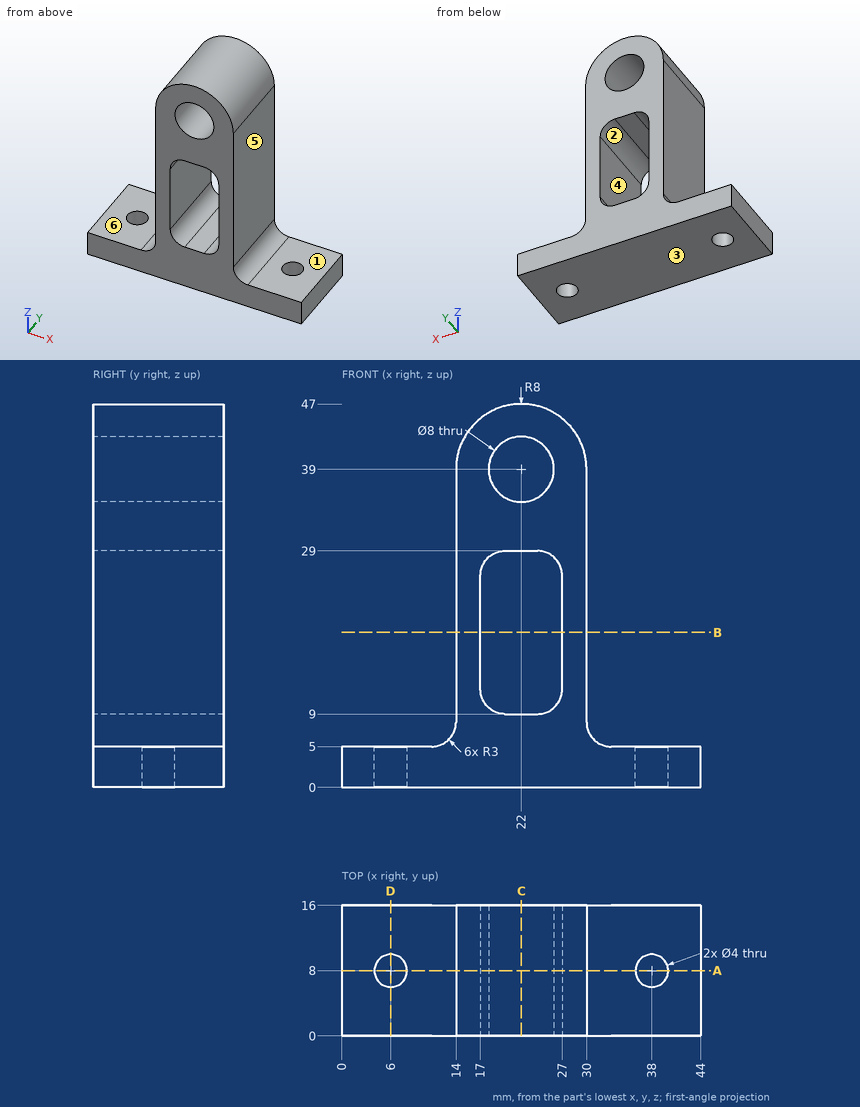
Geometry: see drawing. Coordinates: mm, zero at the bounding-box minimum. A direction names the side the tool comes from. Coordinates: 2 decimals unless noted, no trailing zeros. Loops run counter-clockwise (first coordinate to the right, second up) from the corner with the lowest first, then second, coordinate; pieces in that order, holes last.
(1) Section D-D on x = 6. Return the cut outline in (y, z), then the cut area to 3 significant figures.
(2) First-contact query: pin 1 Ø2 at (x, y) = (34.5, 8) entering from +Z; pin 2 Ø8 at (x, y) = (32.5, 10) entering from +Z; pin 3 Ø7 at (y, z) = (4, 20) entering from -X. Flat tips, straight axial feed; report the tip coordinate or a pass-through.
(3) Section A-A on y = 8. Return the cut outline in (x, z).
(4) Set-up query: the marked faces 4, 5 and 6. Return all of +Z, -Z, +X, -X, +Y, -Y with unobstructed straight access to the full face (end or side cutting, diameter ignored); none if empty.
(5) Pull-direction query (Z, two-part tool) for the marked faces 1, 2 and 3; classes: released by +Z, released by -Z, zero draft, split by the parting line, or undercut.
(6) Section C-C on x = 22. Return the cut outline in (y, z).
(7) Material intervals for probe 1 along X at (y, z) = (8, 2.9); probe 2 along Z at (x, y) = (22, 10.75); probe 3 along X at (y, z) = (9.75, 14), sorted ascending.
(8) Section B-B on z = 19. Return the cut outline in (x, y).
Data:
1. outline: (0, 0) - (6, 0) - (6, 5) - (0, 5) - close; (10, 0) - (16, 0) - (16, 5) - (10, 5) - close
1. area: 60.0 mm2
2. pin 1: stops at z = 5
2. pin 2: stops at z = 43.66
2. pin 3: stops at x = 14
3. outline: (0, 0) - (4, 0) - (4, 5) - (0, 5) - close; (8, 0) - (36, 0) - (36, 5) - (33, 5) arc R3 cw to (30, 8) - (30, 39) arc R8 ccw to (14, 39) - (14, 8) arc R3 cw to (11, 5) - (8, 5) - close; (40, 0) - (44, 0) - (44, 5) - (40, 5) - close; hole (17, 12) arc R3 ccw to (20, 9) - (24, 9) arc R3 ccw to (27, 12) - (27, 26) arc R3 ccw to (24, 29) - (20, 29) arc R3 ccw to (17, 26) - close; hole circle Ø8 at (22, 39)
4. face 4: +Y, -Y
4. face 5: +Z, +X, +Y, -Y
4. face 6: +Z, -X, +Y, -Y
5. face 1: released by +Z
5. face 2: undercut
5. face 3: released by -Z
6. outline: (0, 0) - (16, 0) - (16, 9) - (0, 9) - close; (0, 29) - (16, 29) - (16, 35) - (0, 35) - close; (0, 43) - (16, 43) - (16, 47) - (0, 47) - close
7. probe 1: x = 0 to 4, 8 to 36, 40 to 44
7. probe 2: z = 0 to 9, 29 to 35, 43 to 47
7. probe 3: x = 14 to 17, 27 to 30
8. outline: (14, 0) - (17, 0) - (17, 16) - (14, 16) - close; (27, 0) - (30, 0) - (30, 16) - (27, 16) - close
